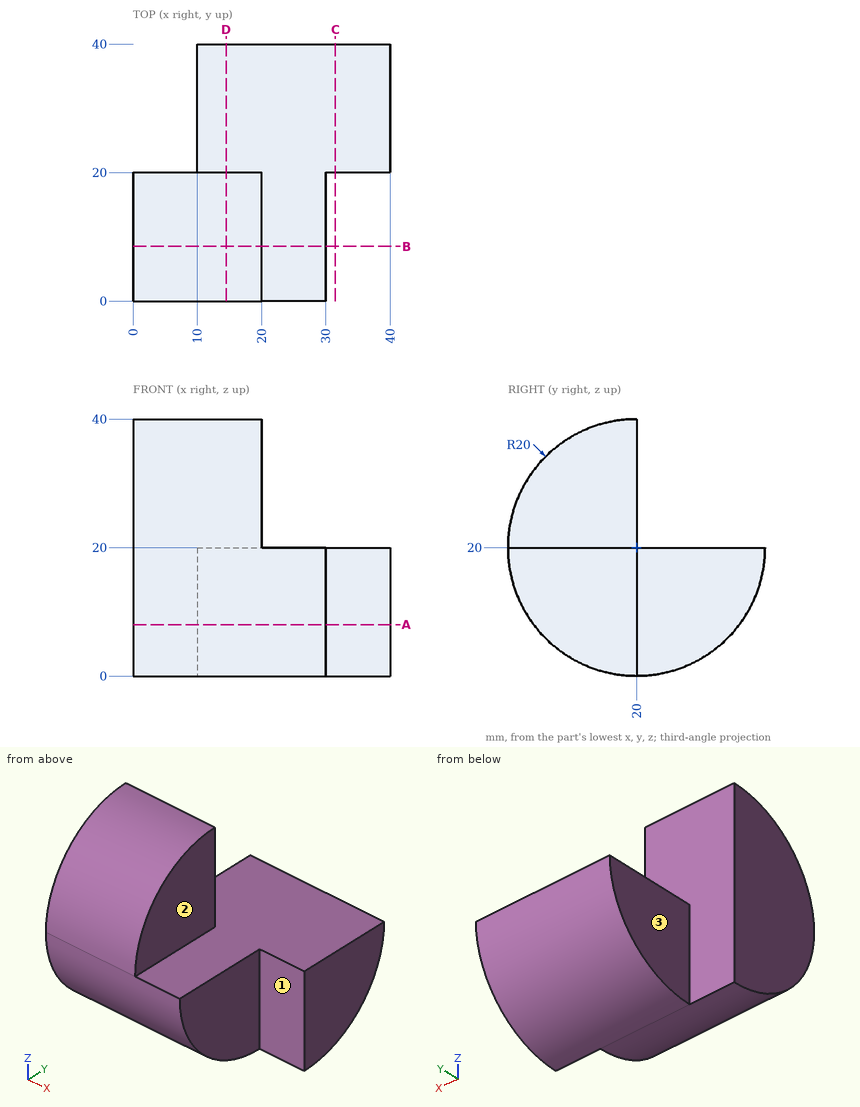
Part print with two shaded views. Sizes in mm from the minimum x, y, z corner. A direction names the side the tool comes from. Round coordinates to 2 decimals unless told otherwise and drop trailing zeros. Write each loop counter-clockwise with the first axis right and the second up, starting at its lowest first coordinate (ties: lowest second). Pieces come first, ordered by that corner, then holes. Notation, with made-up numbers: (41.25, 82) - (89.25, 82) arc R14 cw to (89.25, 96) - close; hole circle Ø2 at (5.5, -9.75). An arc over 180 degrees is marked (long way). Use CSV: the item, a comma, the result in double quotes.
Item 1: Slice it at D-D, the plane x = 14.5. Write the cut outline in (y, z), then the cut area to 3 significant figures.
Results list:
outline,"(20, 20) - (20, 40) arc R20 ccw (long way) to (40, 20) - close"
area,"942 mm²"
Item 2: Wall check: L1, parallel to X at y = 8, z = 17; L2, parallel to X at y = 23.5, z = 18.5; L3, parallel to Z at x = 29, y = 19. Give the ranges that are in metal, low to high.
Results list:
L1,"x = 0 to 30"
L2,"x = 10 to 40"
L3,"z = 0.03 to 20"
Item 3: Slice it at A-A, the plane z = 8. Write the cut outline in (x, y), then the cut area to 3 significant figures.
Results list:
outline,"(0, 4) - (30, 4) - (30, 20) - (40, 20) - (40, 36) - (10, 36) - (10, 20) - (0, 20) - close"
area,"960 mm²"
Item 4: Slice it at C-C, the plane x = 31.5. Write the cut outline in (y, z), then the cut area to 3 significant figures.
Results list:
outline,"(20, 0) arc R20 ccw to (40, 20) - (20, 20) - close"
area,"314 mm²"
Item 5: Slice it at B-B, the plane y = 8.5. Write the cut outline in (x, z), then the cut area to 3 significant figures.
Results list:
outline,"(0, 3.64) - (30, 3.64) - (30, 20) - (20, 20) - (20, 36.36) - (0, 36.36) - close"
area,"818 mm²"
Item 6: Flat gauge pins, fed straight in: P1, Ø6, axis at x = 14.5, z = 14, coming from the +Y side; P2, Ø16, axis at y = 14.5, z = 6, coming from the +X side; P3, Ø1, axis at x = 21.5, y = 24.5, coming from the +Z side; P4, Ø6, axis at y = 25, z = 27.5, coming from the -X side. Where does each tip first touch, or does it go through?
Results list:
P1,"stops at y = 39.77"
P2,"stops at x = 40"
P3,"stops at z = 20"
P4,"passes through"
Item 7: Tool access for the marked faces 1, 2 and 3: list every direction of +Z, -Z, +X, -X, +Y, -Y with a clear straight run to the whole face (end or side of a thin tool).
Results list:
face 1,"+Z, -Z, +X, -Y"
face 2,"+Z, +X, +Y, -Y"
face 3,"+Z, -Z, -X, +Y"
